```python
from build123d import *

# Parameters (mm, degrees)
SKETCH_1_W          = 15
SKETCH_1_H          = 29
SKETCH_1_R          = 1.25
EXTRUDE_1_DEPTH     = 4
SKETCH_2_R          = 1.95
CUT_EXTRUDE_1_DEPTH = 2
CHAMFER_1_SIZE      = 1


with BuildPart() as part:
    # Эскиз1 → Бобышка-Вытянуть1 (new body)
    with BuildSketch(Plane(origin=(0, 0, 0), x_dir=(0, 0, -1), z_dir=(1, 0, 0))):
        Rectangle(SKETCH_1_W, SKETCH_1_H)
        with Locations((0, 6)):
            Circle(SKETCH_1_R, mode=Mode.SUBTRACT)
        with Locations(Location((0, -6, 0), (0, 0, 180))):
            Circle(SKETCH_1_R, mode=Mode.SUBTRACT)
    extrude(amount=EXTRUDE_1_DEPTH)

    # Эскиз2 → Вырез-Вытянуть1 (cut)
    with BuildSketch(Plane(origin=(4, 0, 0), x_dir=(0, 0, -1), z_dir=(1, 0, 0))):
        with Locations((0, 6)):
            Circle(SKETCH_2_R)
        with Locations((0, -6)):
            Circle(SKETCH_2_R)
    extrude(amount=-CUT_EXTRUDE_1_DEPTH, mode=Mode.SUBTRACT)

    # Фаска1
    chamfer_1_edges = [part.edges().sort_by_distance(p)[0] for p in [
        (4, -14.5, 0),
        (4, 14.5, 0),
    ]]
    chamfer(chamfer_1_edges, length=CHAMFER_1_SIZE)


solid = part.part
```
Could you check a few things on this model? Use its own coordinates, in mm. A direction names the side the tool comes from. Coordinates: 2 decimals unless noted, no trailing zeros. Order: outer loops, then holes, each group sorted by start corner. A loop starts at its lowest first (then second) coordinate and runs counter-clockwise, first axis right, second up. Notation, with made-up numbers: M 42,63 L 55,63 A10 cw 55,79 Z; hole C 47,18 d4. An arc over 180 degrees is marked long. Use one line per item in the form item = value. Start each with the question number.
1. Suppose I cut it at A-A on x = 1.2. Write out the boundary of the cut face in (y, z).
2. On a 3-axis mill with a long thin cutter (end or side, diameter ignored), from which of +Z, -Z, +X, -X, +Y, -Y can I reach the whole of each face in a straight line? I mean faces 5 (the flat face through (3.5, -14, 0.1)), 6 (the cylindrical face through (3.014, 7.933, 0.254)). Say none if no direction works.
3. For pin 1 (6 mm diameter, centred on y = 3, z = 2, fed in from -X), with a flat end and sliding along its axis, tell me the tip position at first contact or that it passes through.
4. Suppose I cut it at C-C on y = -6. Write out the boundary of the cut face in (x, z), then the cut area to 3 significant figures.
5. Please list where these lines run through material, in increasing order: line 1 (Y direction, x = 0.85, z = 0); line 2 (Z direction, x = 1.35, y = 6); line 3 (Y direction, x = 3.45, z = 0).
6. Suppose I cut it at B-B on z = 0. Write out the boundary of the cut face in (x, y), then the cut area to 3 significant figures.
7. Suppose I cut it at D-D on x = 2.65. Write out the boundary of the cut face in (y, z).
8. We'd pull the mould along Z, two halves only. Please class faces 1 (the flat face through (4, 0, 0)), 2 (the flat face through (2, 7, 1)), 3 (the flat face through (2, 0, 7.5)), 4 (the flat face through (2, -5, 1)): +Z half, -Z half, draft (parallel to the pull), parting line (faces both ways), or undercut.
Geometry says:
q1.outline = M -14.5,-7.5 L 14.5,-7.5 L 14.5,7.5 L -14.5,7.5 Z; hole C -6,0 d2.5; hole C 6,0 d2.5
q2.face_5 = +Z, -Z, +X, -Y
q2.face_6 = +X
q3.pin_1 = 0
q4.outline = M 0,-7.5 L 4,-7.5 L 4,-1.95 L 2,-1.95 L 2,-1.25 L 0,-1.25 Z; M 0,1.25 L 2,1.25 L 2,1.95 L 4,1.95 L 4,7.5 L 0,7.5 Z
q4.area = 47.2 mm^2
q5.line_1 = -14.5 to -7.25, -4.75 to 4.75, 7.25 to 14.5
q5.line_2 = -7.5 to -1.25, 1.25 to 7.5
q5.line_3 = -14.05 to -7.95, -4.05 to 4.05, 7.95 to 14.05
q6.outline = M 0,-14.5 L 3,-14.5 L 4,-13.5 L 4,-7.95 L 2,-7.95 L 2,-7.25 L 0,-7.25 Z; M 0,-4.75 L 2,-4.75 L 2,-4.05 L 4,-4.05 L 4,4.05 L 2,4.05 L 2,4.75 L 0,4.75 Z; M 0,7.25 L 2,7.25 L 2,7.95 L 4,7.95 L 4,13.5 L 3,14.5 L 0,14.5 Z
q6.area = 89.4 mm^2
q7.outline = M -14.5,-7.5 L 14.5,-7.5 L 14.5,7.5 L -14.5,7.5 Z; hole C -6,0 d3.9; hole C 6,0 d3.9
q8.face_1 = draft
q8.face_2 = undercut
q8.face_3 = +Z half
q8.face_4 = undercut
